from build123d import *

# Parameters (mm, degrees)
F0_W     = 25.4
F0_H     = 6.35
F1_DEPTH = 6.35


with BuildPart() as f1:
    # F0 (on Top) → F1 (new body)
    with BuildSketch(Plane.XY):
        Polygon((-171.398427, 22), (-171.398427, 0), (-145.998427, 0), (-120.598427, 0), (-12.7, 0), (12.7, 0), (120.598427, 0), (145.998427, 0), (171.398427, 0), (171.398427, 22), (127.028518, 15.766784), (101.875509, 12.233216), (57.5056, 6), (12.7, 6), (-12.7, 6), (-57.5056, 6), (-101.875509, 12.233216), (-127.028518, 15.766784), align=None)
        with Locations((-133.298427, -3.175)):
            Rectangle(F0_W, F0_H)
        Polygon((-126.145126, 22.055037), (-127.028518, 15.766784), (-101.875509, 12.233216), (-100.992117, 18.521468), align=None)
        with Locations((0, -3.175)):
            Rectangle(F0_W, F0_H)
        with Locations((133.298427, -3.175)):
            Rectangle(F0_W, F0_H)
        with Locations((0, 9.175)):
            Rectangle(F0_W, F0_H)
        Polygon((100.992117, 18.521468), (101.875509, 12.233216), (127.028518, 15.766784), (126.145126, 22.055037), align=None)
    extrude(amount=F1_DEPTH)


solid = f1.part
The listing builds one solid part. Answer for the finished solid, in the listing's coordinates (mm). A direction names the side the tool comes from. Give positions to 0.01 mm unless a question says otherwise; leave off trailing zeros. Write each loop counter-clockwise with the first axis right and the second up, starting at its lowest first coordinate (ties: lowest second). Pieces come first, ordered by that corner, then holes.
1) Find the intervals of material crossed by L1, parallel to X at y = -4, z = 2.5; L2, parallel to X at y = 13.5, z = 1.75; L3, parallel to Y at x = 10, z = 6, in increasing order.
2) Section C-C (x = -32) is taken. Write down the section's boundary in (y, z), and give its area (3 significant figures).
3) Given P1, Ø1.9, axis at y = -2, z = 3, coming from the -X side; P2, Ø1.9, axis at x = -92, z = 2, coming from the -Y side; P3, Ø3, axis at x = -33.5, z = 3, coming from the +Y side; P4, Ø4, axis at x = 0.5, y = 10, coming from the -Z side, each flat-ended and moving along its own axis, determine where each tip first touches the part or whether it passes through.
4) Section D-D (x = 70) is taken. Write down the section's boundary in (y, z).
5) A tool of negligible diameter and unlimited length cuts with its end or side. For faces 1 (the face through (113.745, 20.313, 3.131)), 2 (the face through (159, 0, 3)), 3 (the face through (12.7, -3, 3)), 4 (the face through (133, -6.35, 3)), 5 (the face through (101.428, 15.421, 3.131)), from which of +Z, -Z, +X, -X, +Y, -Y can it reach the whole face along a straight path? Write none if from no direction.
6) Section A-A (y = -3) is taken. Write down the section's boundary in (x, z), and give its area (3 significant figures).
7) For a pull along X with two mould halves and no side action, classify faces 6 (the face through (-171.398, 11, 3)), 7 (the face through (-159, 0, 3)), 8 (the face through (80, 9.16, 3.13)) as pulls with the +X half, pulls with the -X half, needs draft (parallel to the pull), parting line crosses it, or undercut.
Response:
1. L1: x = -146 to -120.6, -12.7 to 12.7, 120.6 to 146
1. L2: x = -171.4 to -101.7, 101.7 to 171.4
1. L3: y = -6.35 to 12.35
2. outline: (0, 0) - (6, 0) - (6, 6.35) - (0, 6.35) - close
2. area: 38.1 mm2
3. P1: stops at x = -146
3. P2: stops at y = 0
3. P3: stops at y = 6
3. P4: stops at z = 0
4. outline: (0, 0) - (7.76, 0) - (7.76, 6.35) - (0, 6.35) - close
5. face 1: +Z, -Z, +Y
5. face 2: +Z, -Z, +X, -Y
5. face 3: +Z, -Z, -Y
5. face 4: +Z, -Z, +X, -X, -Y
5. face 5: +Z, -Z
6. outline: (-146, 0) - (-120.6, 0) - (-120.6, 6.35) - (-146, 6.35) - close; (-12.7, 0) - (12.7, 0) - (12.7, 6.35) - (-12.7, 6.35) - close; (120.6, 0) - (146, 0) - (146, 6.35) - (120.6, 6.35) - close
6. area: 484 mm2
7. face 6: pulls with the -X half
7. face 7: needs draft
7. face 8: undercut
